```python
from build123d import *

# Parameters (mm, degrees)
F0_W           = 107.2001978755
F0_H           = 86.5053012967
F1_DEPTH       = 100
F3_D           = 15
F3_CBORE_D     = 25
F3_CBORE_DEPTH = 50
F4_T           = -2.5


with BuildPart() as f1:
    # F0 (on Front) → F1 (new body)
    with BuildSketch(Plane.XZ):
        with Locations((-2.1000653505, -2.4665594101)):
            Rectangle(F0_W, F0_H)
    extrude(amount=-F1_DEPTH)

    # F3 (through all)
    with Locations(Plane.XY.offset(40.7860912383)):
        with Locations((9.1865165159, 57.8404814005)):
            CounterBoreHole(F3_D / 2, F3_CBORE_D / 2, F3_CBORE_DEPTH)

    # F4
    f4_openings = [f1.faces().sort_by_distance(p)[0] for p in [
        (-2.641683, 49.623753, 40.786091),
    ]]
    offset(amount=F4_T, openings=f4_openings, kind=Kind.INTERSECTION)


solid = f1.part
```
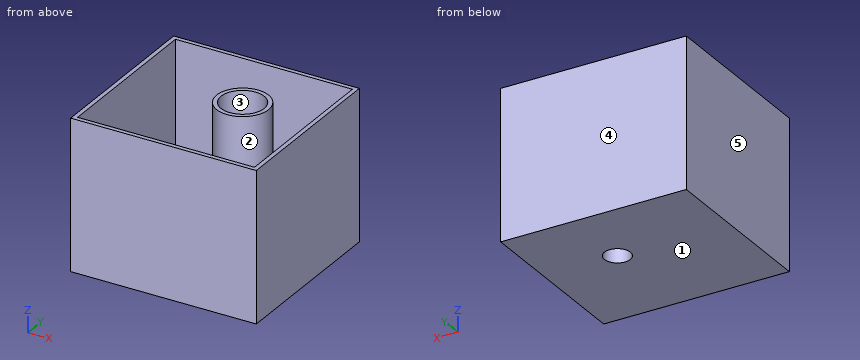
Part model, mm, in its own coordinate system. Face numbers are marked on the shaded views. A direction names the side the tool comes from. Round coordinates to 2 decimals unless told otherwise and drop trailing zeros. Write each loop counter-clockwise with the first axis right and the second up, starting at its lowest first coordinate (ties: lowest second). Pieces come first, ordered by that corner, then holes.
Item 1: Which spindle directions (+Z, -Z, +X, -X, +Y, -Y) get a long thin tool onto all of the face, cutting with end or side? Do the marked faces 1 and 2. Say none if no direction does.
Results:
face 1: -Z, +X, -X, +Y, -Y
face 2: +Z
Item 2: Probe L1, parallel to Y at x = -45.5, z = 8.5; L2, parallel to X at y = 16.5, z = -14; L3, parallel to Y at x = 15, z = -27.5. List the from-to ranges inside material, lowest first.
Results:
L1: y = 0 to 2.5, 97.5 to 100
L2: x = -55.7 to -53.2, 49 to 51.5
L3: y = 0 to 2.5, 49.7 to 53.1, 62.58 to 65.98, 97.5 to 100
Item 3: Cut at D-D, the plane y = 26.5. Give the cut face in (x, z), plus the area to 3 significant figures.
Results:
outline: (-55.7, -45.72) - (51.5, -45.72) - (51.5, 40.79) - (49, 40.79) - (49, -43.22) - (-53.2, -43.22) - (-53.2, 40.79) - (-55.7, 40.79) - close
area: 688 mm2
Item 4: Cut at A-A, the plane z = -15. Give the cut face in (x, y), plus the area to 3 significant figures.
Results:
outline: (-55.7, 0) - (51.5, 0) - (51.5, 100) - (-55.7, 100) - close; circle Ø20 at (9.19, 57.84); hole (-53.2, 2.5) - (49, 2.5) - (49, 97.5) - (-53.2, 97.5) - close; hole circle Ø15 at (9.19, 57.84)
area: 1,150 mm2
Item 5: Two-plate mould, pull along Y, no slides. Class the marked faces 3, 4 and 5: +Y half, -Y half, draft (parallel to the pull), parting line (faces both ways), or undercut.
Results:
face 3: undercut
face 4: +Y half
face 5: draft
Item 6: Cut at B-B, the plane y = 53.5. Give the cut face in (x, z).
Results:
outline: (-55.7, -45.72) - (3.07, -45.72) - (3.07, -9.21) - (-2.54, -9.21) - (-2.54, 40.79) - (-5.17, 40.79) - (-5.17, -11.71) - (0.18, -11.71) - (0.18, -43.22) - (-53.2, -43.22) - (-53.2, 40.79) - (-55.7, 40.79) - close; (15.3, -45.72) - (51.5, -45.72) - (51.5, 40.79) - (49, 40.79) - (49, -43.22) - (18.2, -43.22) - (18.2, -11.71) - (23.54, -11.71) - (23.54, 40.79) - (20.91, 40.79) - (20.91, -9.21) - (15.3, -9.21) - close
Item 7: Drop flat-ended pins along their axis: pin 1 Ø4 at (x, y) = (-39, 62) entering from +Z; pin 2 Ø22.5 at (x, y) = (9.19, 57.84) entering from +Z. Give the stop position or say it passes through.
Results:
pin 1: stops at z = -43.22
pin 2: stops at z = -9.21
Item 8: Cut at C-C, the plane x = -44. Give the cut face in (y, z), plus the area to 3 significant figures.
Results:
outline: (0, -45.72) - (100, -45.72) - (100, 40.79) - (97.5, 40.79) - (97.5, -43.22) - (2.5, -43.22) - (2.5, 40.79) - (0, 40.79) - close
area: 670 mm2
